For this review, take the finished solid that the model builds, in its own axes (mm). Face numbers are marked on the shaded views. Round coordinates to 2 decimals unless told otherwise and drop trailing zeros. Loops run counter-clockwise (first coordinate to the right, second up) from the corner with the lowest first, then second, coordinate; pieces in that order, holes last.
1) Wall thickness on L1, parallel to Y at x = 0, z = -0.7 (3 decimals); L2, parallel to Y at x = -2, z = -1; L3, parallel to Z at x = 3, y = -1 (3 decimals): over which ranges is each line inside the solid? List them lowest first.
2) Take a section at A-A (z = -8). State the section outline as (x, y) points (3 decimals), then the cut area to 3 significant figures.
3) Insertion check: pin 1 (2 mm diameter, centred on x = -2, z = -6, fed in from +Y); pin 2 (2 mm diameter, centred on x = -9.5, z = -5.5, fed in from +Y); pin 3 (4.5 mm diameter, centred on x = 1, y = 0, fed in from +Z) (3 decimals). Each pin has a flat end and moves straight along its axis. Give the tip position at first contact, or say it passes through.
4) Mouldability with a two-part tool opening along Y and no side actions: class the marked faces 1, 2, 3 and 4 as pulls with the +Y half, pulls with the -Y half, needs draft (parallel to the pull), parting line crosses it, or undercut.
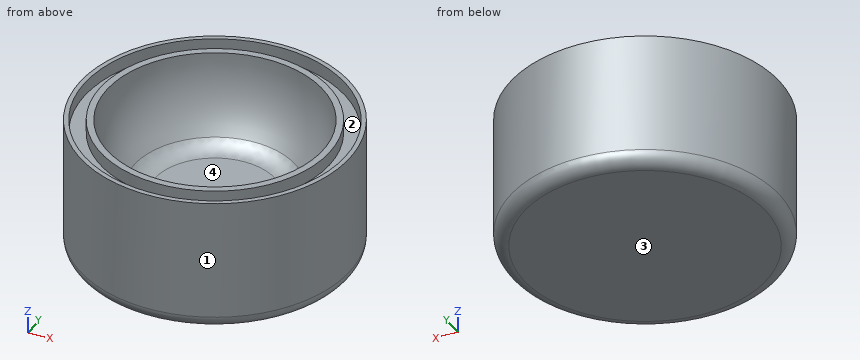
```python
from build123d import *

# Parameters (mm, degrees)
F2_DEPTH = 6.35
F3_R     = 3.175
F4_R     = 15.33125
F4_R_2   = 13.49375
F5_DEPTH = 1.5875
F6_R     = 1.5875


with BuildPart() as f1:
    # F0 (on Front) → F1 (revolve)
    with BuildSketch(Plane.XZ):
        with BuildLine():
            Line((0, -15.875), (0, -12.7))
            ThreePointArc((0, -12.7), (-8.9802561211, -8.9802561211), (-12.7, 0))
            Line((-12.7, 0), (-15.875, 0))
            Line((-15.875, 0), (-15.875, -15.875))
            Line((-15.875, -15.875), (0, -15.875))
        make_face()
    revolve(axis=Axis((0, 0, -1.4379415661), (0, 0, -1)))

    # F2 (add): a face of the model
    f2_faces = [f1.faces().sort_by_distance(p)[0] for p in [
        (0, 0, -15.875),
    ]]
    extrude(f2_faces, amount=-F2_DEPTH)

    # F3
    f3_edges = [f1.edges().sort_by_distance(p)[0] for p in [
        (8.40026, 0, -9.525),
    ]]
    fillet(f3_edges, radius=F3_R)

    # F4 (on face) → F5 (cut)
    with BuildSketch(Plane.XY):
        Circle(F4_R)
        Circle(F4_R_2, mode=Mode.SUBTRACT)
    extrude(amount=-F5_DEPTH, mode=Mode.SUBTRACT)

    # F6
    f6_edges = [f1.edges().sort_by_distance(p)[0] for p in [
        (15.875, 0, -15.875),
    ]]
    fillet(f6_edges, radius=F6_R)


solid = f1.part
```
Response:
1. L1: y = -15.875 to -15.331, -13.494 to -12.681, 12.681 to 13.494, 15.331 to 15.875
1. L2: y = -15.75 to -15.2, -13.34 to -12.5, 12.5 to 13.34, 15.2 to 15.75
1. L3: z = -15.875 to -9.525
2. outline: circle Ø31.75 at (0, 0); hole circle Ø19.727 at (0, 0)
2. area: 486 mm2
3. pin 1: stops at y = 15.84
3. pin 2: stops at y = 13.41
3. pin 3: stops at z = -9.525
4. face 1: parting line crosses it
4. face 2: undercut
4. face 3: needs draft
4. face 4: undercut
